Model file for the job. Use its own axes, mm. Face numbers are marked on the shaded views. Round coordinates to 2 decimals unless told otherwise and drop trailing zeros. Order: outer loops, then holes, each group sorted by start corner. A loop starts at its lowest first (then second) coordinate and runs counter-clockwise, first axis right, second up. Notation, with made-up numbers: (76, 66) -> (112, 66) arc R27 ccw to (112, 91) -> close; hole circle Ø2 at (15.25, 24). An arc over 180 degrees is marked (long way). Use CSV: the item, a comma, the result in double quotes.
```python
from build123d import *

# Parameters (mm, degrees)
SKETCH1_R             = 19.05
SKETCH1_R_2           = 12.4206
BOSS_EXTRUDE1_DEPTH   = 4.3688
SKETCH4_R             = 19.05
SKETCH4_R_2           = 13.462
BOSS_EXTRUDE2_DEPTH   = 0.889
F_4_CLEARANCE_HOLE1_D = 3.2639
CHAMFER1_SIZE         = 0.1524
CHAMFER2_SIZE         = 0.508


with BuildPart() as part:
    # Sketch1 → Boss-Extrude1 (new body)
    with BuildSketch(Plane.XY):
        with Locations((-8.514490438, 61.389045102)):
            Circle(SKETCH1_R)
        with Locations((-8.514490438, 61.389045102)):
            Circle(SKETCH1_R_2, mode=Mode.SUBTRACT)
    extrude(amount=BOSS_EXTRUDE1_DEPTH)

    # Sketch4 → Boss-Extrude2 (add)
    with BuildSketch(Plane(origin=(0, 0, 0), x_dir=(-1, 0, 0), z_dir=(0, 0, -1))):
        with Locations((8.514490438, 61.389045102)):
            Circle(SKETCH4_R)
        with Locations((8.514490438, 61.389045102)):
            Circle(SKETCH4_R_2, mode=Mode.SUBTRACT)
    extrude(amount=BOSS_EXTRUDE2_DEPTH)

    # #4 Clearance Hole1 (through all)
    with Locations(Plane(origin=(-12.913159706, 9.247820606, 4.3688), x_dir=(1, 0, 0), z_dir=(0, 0, 1))):
        with Locations((17.596896421, 59.80259772), (-8.799557886, 59.80259772), (4.398669267, 36.94259772)):
            Hole(F_4_CLEARANCE_HOLE1_D / 2)

    # Chamfer1
    chamfer1_edges = [part.edges().sort_by_distance(p)[0] for p in [
        (-20.935090438, 61.389045102, 0),
    ]]
    chamfer(chamfer1_edges, length=CHAMFER1_SIZE)

    # Chamfer2
    chamfer2_edges = [part.edges().sort_by_distance(p)[0] for p in [
        (-27.564490438, 61.389045102, 4.3688),
    ]]
    chamfer(chamfer2_edges, length=CHAMFER2_SIZE)


solid = part.part
```
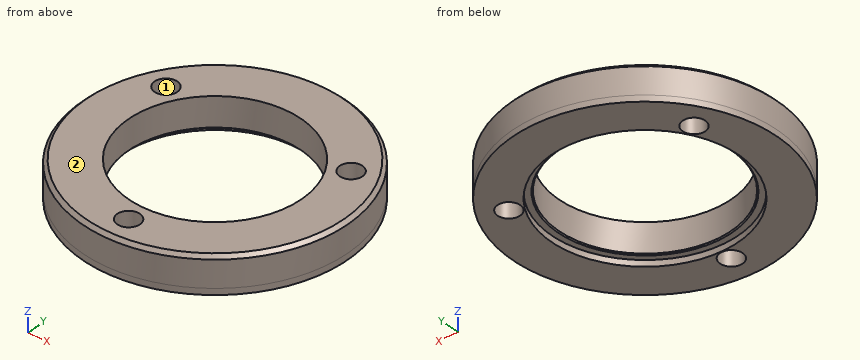
Q1. Mould opens along X. For the marked faces 1 and 2 say: +X half, -X half, draft (parallel to the pull), parting line (faces both ways), or undercut.
From the geometry:
face 1,"undercut"
face 2,"draft"
Q2. Probe line 1 along X through (y, z) = (61.5, 2.9); line 2 along Y through (x, z) = (-10, 3.55); line 3 along Y through (x, z) = (2.5, 1.35). List the from-to ranges inside material, lowest first.
From the geometry:
line 1,"x = -27.56 to -20.93, 3.91 to 10.54"
line 2,"y = 42.4 to 45.51, 46.87 to 49.06, 73.72 to 80.38"
line 3,"y = 45.85 to 55.65, 67.13 to 76.93"
Q3. Pin check, flat tips, straight feed: pin 1 (2 mm diameter, centred on x = -1.5, z = 3.5, fed in from -Y); pin 2 (4 mm diameter, centred on x = -21.71, y = 69.05, fed in from +Z); pin 3 (1 mm diameter, centred on x = -10, z = 3.5, fed in from -Y); pin 4 (2 mm diameter, centred on x = -15, z = 3.5, fed in from -Y). Stop position of each tip, or through.
From the geometry:
pin 1,"stops at y = 43.31"
pin 2,"stops at z = 4.37"
pin 3,"stops at y = 42.36"
pin 4,"stops at y = 43.15"
Q4. Cut at A-A (z = 3.3). Give the cut face in (x, y), plus the area to 3 significant figures.
From the geometry:
outline,"circle Ø38.1 at (-8.51, 61.39); hole circle Ø3.26 at (-21.71, 69.05); hole circle Ø24.84 at (-8.51, 61.39); hole circle Ø3.26 at (-8.51, 46.19); hole circle Ø3.26 at (4.68, 69.05)"
area,"630 mm²"
